Work out the finished part from the listing and answer in its coordinate system (mm). A direction names the side the tool comes from. Give positions to 0.01 mm unless a question says otherwise; leave off trailing zeros. Loops run counter-clockwise (first coordinate to the right, second up) from the corner with the lowest first, then second, coordinate; pieces in that order, holes last. Notation, with made-up numbers: (48, -10) -> (78, -10) arc R30 cw to (78, 20) -> close; hole circle Ø11 at (-1, 69.25). An arc over 180 degrees is marked (long way). Answer as CSV lines item,"result". Start each with the question number.
1. Flat-ended cylindrical pins translate along their axes: pin 1 Ø8 at (x, y) = (-13.5, 7.5) entering from +Z; pin 2 Ø5 at (y, z) = (15, -3) entering from -X; pin 3 Ø6 at (y, z) = (11.5, 13) entering from -X. Find the tip coordinate at first contact, or state that the pin passes through.
2. Find section D-D, the plane y = 14. Give the vertices of the cut face in (x, z), and give its area (3 significant figures).
3. Find the intervals of material crossed by line 1 along Z through (x, y) = (-12.5, 4); line 2 along Y through (x, z) = (-14, 1); line 3 along Y through (x, z) = (9, -1), in increasing order.
4. Determine the mould class of faces 1 (the face through (16.5, 16, 0)), 2 (the face through (-2.343, 8.381, -17.847)), 3 (the face through (0, 17, -4)) for opening direction Z: +Z half, -Z half, draft (parallel to the pull), parting line (faces both ways), or undercut.
5. Find section B-B, the plane z = 0. Give the vertices of the cut face in (x, y).
6. Find section A-A, the plane y = 1.5. Give the vertices of the cut face in (x, z), and give its area (3 significant figures).
7. A tool of negligible diameter and unlimited length cuts with its end or side. For faces 4 (the face through (0, 0, 8)), 5 (the face through (13, 3, 0)), 6 (the face through (-16.5, 16, 0)), from which of +Z, -Z, +X, -X, +Y, -Y can it reach the whole face along a straight path? Write none if from no direction.
8. Find section C-C, the plane x = 5.5. Give the vertices of the cut face in (y, z), and give its area (3 significant figures).
from build123d import *

# Parameters (mm, degrees)
SKETCH1_R           = 18
BOSS_EXTRUDE1_DEPTH = 17
SKETCH2_W           = 26
SKETCH2_H           = 14
CUT_EXTRUDE1_DEPTH  = 5.25
CUT_EXTRUDE2_DEPTH  = 2


with BuildPart() as part:
    # Sketch1 → Boss-Extrude1 (new body)
    with BuildSketch(Plane(origin=(0, 0, 0), x_dir=(1, 0, 0), z_dir=(0, 1, 0))):
        Circle(SKETCH1_R)
    extrude(amount=BOSS_EXTRUDE1_DEPTH)

    # Sketch2 → Cut-Extrude1 (cut)
    with BuildSketch(Plane.XZ):
        Rectangle(SKETCH2_W, SKETCH2_H)
    extrude(amount=-CUT_EXTRUDE1_DEPTH, mode=Mode.SUBTRACT)

    # Sketch3 → Cut-Extrude2 (cut)
    with BuildSketch(Plane(origin=(0, 17, 0), x_dir=(1, 0, 0), z_dir=(0, 1, 0))):
        with BuildLine():
            Line((14.5, 2), (0.364696883, 3.480947599))
            ThreePointArc((0.364696883, 3.480947599), (0, 3.5), (-0.364696883, 3.480947599))
            Line((-0.364696883, 3.480947599), (-14.5, 2))
            ThreePointArc((-14.5, 2), (-16.5, 0), (-14.5, -2))
            Line((-14.5, -2), (-3.185421861, -3.185421861))
            Line((-3.185421861, -3.185421861), (-2, -14.5))
            ThreePointArc((-2, -14.5), (0, -16.5), (2, -14.5))
            Line((2, -14.5), (3.185421861, -3.185421861))
            Line((3.185421861, -3.185421861), (14.5, -2))
            ThreePointArc((14.5, -2), (16.5, 0), (14.5, 2))
        make_face()
    extrude(amount=-CUT_EXTRUDE2_DEPTH, mode=Mode.SUBTRACT)


solid = part.part
Resolved:
1,pin 1,"stops at z = 15.29"
1,pin 2,"stops at x = -17.99"
1,pin 3,"stops at x = -14.97"
2,outline,"circle Ø36 at (0, 0)"
2,area,"1,020 mm^2"
3,line 1,"z = -12.95 to -7, 7 to 12.95"
3,line 2,"y = 0 to 15"
3,line 3,"y = 5.25 to 15"
4,face 1,"undercut"
4,face 2,"parting line"
4,face 3,"draft"
5,outline,"(-18, 0) -> (-13, 0) -> (-13, 5.25) -> (13, 5.25) -> (13, 0) -> (18, 0) -> (18, 17) -> (16.5, 17) -> (16.5, 15) -> (-16.5, 15) -> (-16.5, 17) -> (-18, 17) -> close"
6,outline,"circle Ø36 at (0, 0); hole (-13, -7) -> (13, -7) -> (13, 7) -> (-13, 7) -> close"
6,area,"654 mm^2"
7,face 4,"+Z, -Z, +X, -X, -Y"
7,face 5,"-Y"
7,face 6,"+Y"
8,outline,"(0, -17.14) -> (17, -17.14) -> (17, -2.94) -> (15, -2.94) -> (15, 2.94) -> (17, 2.94) -> (17, 17.14) -> (0, 17.14) -> (0, 7) -> (5.25, 7) -> (5.25, -7) -> (0, -7) -> close"
8,area,"497 mm^2"
